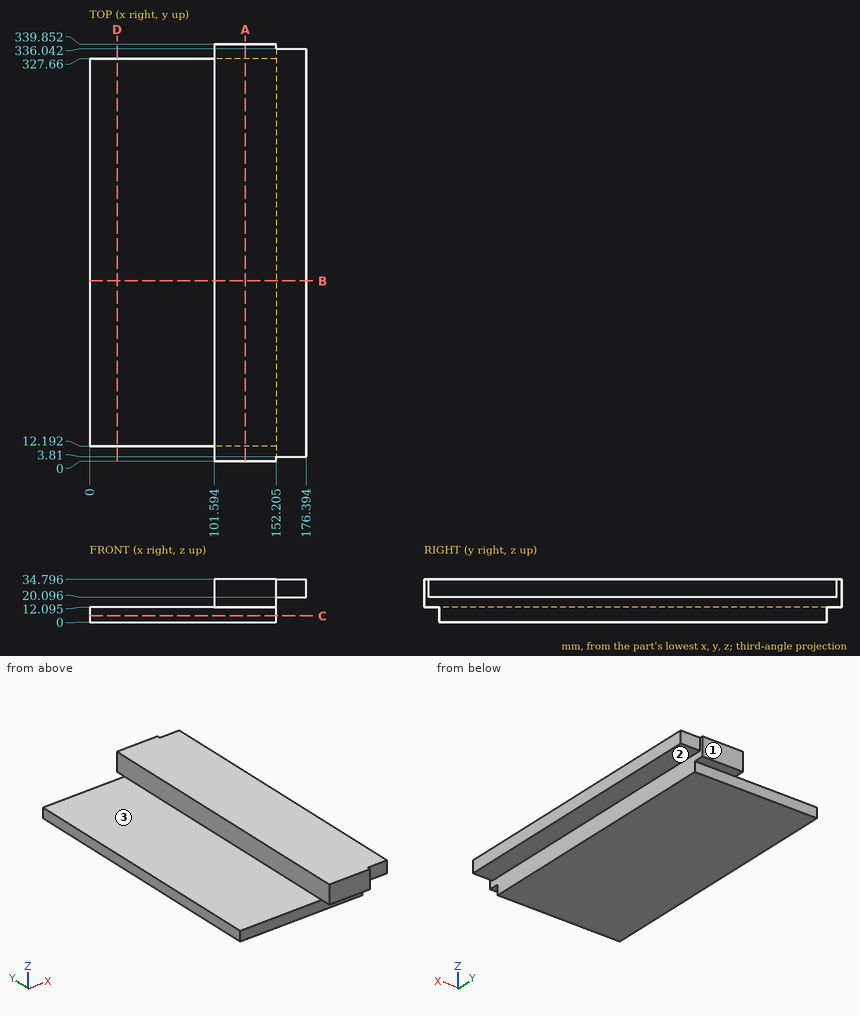
Answer from the drawing. Dimensions are ordinates in mm from the lowest x, y and z of the part. A direction names the side the tool comes from. Coordinates: 2 decimals unless noted, no trailing zeros. Loops run counter-clockwise (first coordinate to the right, second up) from the corner with the lowest first, then second, coordinate; pieces in that order, holes last.
1) Section A-A (x = 127) is taken. Give the vertices of the cut face in (y, z) (1 decimal).
Results:
outline: (0, 12.1) - (12.2, 12.1) - (12.2, 0) - (327.7, 0) - (327.7, 12.1) - (339.9, 12.1) - (339.9, 34.8) - (0, 34.8) - close
2) Section C-C (z = 5) is taken. Give the vertices of the cut face in (x, y) (1 decimal), plus the area to 3 significant figures.
Results:
outline: (0, 12.2) - (152.2, 12.2) - (152.2, 327.7) - (0, 327.7) - close
area: 48,000 mm2
3) Flat-ended cylindrical pins translate along their axes: pin 1 (1 mm diameter, centred on y = 169, z = 11.5, fed in from +X) (1 decimal); pin 2 (3.5 mm diameter, centred on x = 114.5, y = 335.5, fed in from -Z) (3 decimals); pin 3 (1.5 mm diameter, centred on y = 158.5, z = 16, fed in from -X). Find the tip coordinate at first contact, or state that the pin passes through.
Results:
pin 1: stops at x = 152.2
pin 2: stops at z = 12.095
pin 3: stops at x = 101.59
4) Consider probe 1 along X at (y, z) = (86.5, 12.5) (1 decimal); probe 2 along Z at (x, y) = (159, 139); probe 3 along X at (y, z) = (217, 10.5) (1 decimal). Determine where each line is inside the solid, lowest interval first.
Results:
probe 1: x = 101.6 to 152.2
probe 2: z = 20.1 to 34.8
probe 3: x = 0 to 152.2
5) For the marked faces 1, 2 and 3, determine the directions among +Z, -Z, +X, -X, +Y, -Y from which every point of the face is accessible in a straight line to the end or side of a thin tool.
Results:
face 1: +Z, -Z, +X, -X, +Y
face 2: -Z, +X, +Y, -Y
face 3: +Z, -X, +Y, -Y
6) Section B-B (y = 147) is taken. Give the vertices of the cut face in (x, z) (1 decimal).
Results:
outline: (0, 0) - (152.2, 0) - (152.2, 20.1) - (176.4, 20.1) - (176.4, 34.8) - (101.6, 34.8) - (101.6, 12.1) - (0, 12.1) - close
7) Section D-D (x = 22.5) is taken. Give the vertices of the cut face in (y, z) (1 decimal).
Results:
outline: (12.2, 0) - (327.7, 0) - (327.7, 12.1) - (12.2, 12.1) - close
